Could you check a few things on this model? Use its own coordinates, in mm. Round coordinates to 2 decimals unless told otherwise and drop trailing zeros. Write each loop counter-clockwise with the first axis right and the second up, starting at its lowest first coordinate (ties: lowest second). Pieces come first, ordered by that corner, then holes. Notation, with made-up numbers: (-1, 86) -> (27, 86) arc R11 cw to (27, 93) -> close; hole circle Ø3 at (33.5, -18). An arc over 180 degrees is marked (long way). Answer in a Markdown table with one row per item.
from build123d import *

# Parameters (mm, degrees)
F0_R     = 11
F1_DEPTH = 6.9088
F2_R     = 0.762


with BuildPart() as f1:
    # F0 (on Top) → F1 (new body)
    with BuildSketch(Plane.XY):
        with BuildLine():
            ThreePointArc((-30.12, -12.990381), (-18.81, -8.92943), (-7.5, -12.990381))
            Line((-7.5, -12.990381), (-15, 0))
            Line((-15, 0), (-7.5, 12.990381))
            ThreePointArc((-7.5, 12.990381), (-18.81, 8.92943), (-30.12, 12.990381))
            Line((-30.12, 12.990381), (-22.62, 0))
            Line((-22.62, 0), (-30.12, -12.990381))
        make_face()
        Polygon((22.62, 0), (30.12, -12.990381), (45.12, -12.990381), (52.62, 0), (45.12, 12.990381), (30.12, 12.990381), align=None)
        with Locations((37.62, 0)):
            Circle(F0_R, mode=Mode.SUBTRACT)
        Polygon((-45.12, -12.990381), (-30.12, -12.990381), (-22.62, 0), (-30.12, 12.990381), (-45.12, 12.990381), (-52.62, 0), align=None)
        with Locations((-37.62, 0)):
            Circle(F0_R, mode=Mode.SUBTRACT)
        Polygon((7.5, -12.990381), (15, 0), (7.5, 12.990381), (-7.5, 12.990381), (-15, 0), (-7.5, -12.990381), align=None)
        Circle(F0_R, mode=Mode.SUBTRACT)
        with BuildLine():
            Line((7.5, 12.990381), (15, 0))
            Line((15, 0), (7.5, -12.990381))
            ThreePointArc((7.5, -12.990381), (18.81, -8.92943), (30.12, -12.990381))
            Line((30.12, -12.990381), (22.62, 0))
            Line((22.62, 0), (30.12, 12.990381))
            ThreePointArc((30.12, 12.990381), (18.81, 8.92943), (7.5, 12.990381))
        make_face()
    extrude(amount=F1_DEPTH)

    # F2
    f2_edges = [f1.edges().sort_by_distance(p)[0] for p in [
        (-37.62, 12.990381, 6.9088),
        (-18.81, 8.92943, 6.9088),
        (0, 12.990381, 6.9088),
        (18.81, 8.92943, 6.9088),
        (48.87, 6.495191, 6.9088),
        (48.87, -6.495191, 6.9088),
        (37.62, -12.990381, 6.9088),
        (18.81, -8.92943, 6.9088),
        (0, -12.990381, 6.9088),
        (-37.62, -12.990381, 6.9088),
        (-48.87, 6.495191, 6.9088),
        (-48.87, -6.495191, 6.9088),
        (-18.81, -8.92943, 6.9088),
        (37.62, 12.990381, 6.9088),
        (18.81, -8.92943, 0),
        (0, -12.990381, 0),
        (-18.81, -8.92943, 0),
        (-37.62, -12.990381, 0),
        (-48.87, -6.495191, 0),
        (-48.87, 6.495191, 0),
        (37.62, -12.990381, 0),
        (48.87, -6.495191, 0),
        (52.62, 0, 3.4544),
        (37.62, 12.990381, 0),
        (18.81, 8.92943, 0),
        (0, 12.990381, 0),
        (-18.81, 8.92943, 0),
        (-37.62, 12.990381, 0),
        (48.87, 6.495191, 0),
    ]]
    fillet(f2_edges, radius=F2_R)


solid = f1.part
1) Imagine slicing it at D-D, the plane x = -41.5. Please give me the cut outline in (y, z), plus the area to 3 significant figures.
Findings:
| item | result |
|---|---|
| outline | (-12.99, 0.76) arc R0.76 ccw to (-12.23, 0) -> (-10.29, 0) -> (-10.29, 6.91) -> (-12.23, 6.91) arc R0.76 ccw to (-12.99, 6.15) -> close; (10.29, 0) -> (12.23, 0) arc R0.76 ccw to (12.99, 0.76) -> (12.99, 6.15) arc R0.76 ccw to (12.23, 6.91) -> (10.29, 6.91) -> close |
| area | 36.8 mm^2 |
2) For pin 1 (3 mm diameter, centred on y = 3.5, z = 1.5, fed in from -X); pin 2 (2 mm diameter, centred on x = 8, y = -5, fed in from +Z); pin 3 (2 mm diameter, centred on y = 4, z = 5, fed in from +X), each with a flat end and sliding along its axis, tell me the tip position at first contact or that it passes through.
Findings:
| item | result |
|---|---|
| pin 1 | stops at x = -51.47 |
| pin 2 | passes through |
| pin 3 | stops at x = 50.89 |
3) Please list where these lines run through material, in increasing order: line 1 (Y direction, x = 0, z = 4.25); line 2 (X direction, y = 0.25, z = 1.5); line 3 (X direction, y = 5.75, z = 1.25).
Findings:
| item | result |
|---|---|
| line 1 | y = -12.99 to -11, 11 to 12.99 |
| line 2 | x = -52.48 to -48.62, -26.62 to -11, 11 to 26.62, 48.62 to 52.46 |
| line 3 | x = -49.3 to -47, -28.24 to -9.38, 9.38 to 28.24, 47 to 49.3 |
4) Imagine slicing it at C-C, the plane y = 5.75. Count the separate pieces of the cut face and the enclosed holes in it, plus the area to 3 significant figures.
Findings:
| item | result |
|---|---|
| separate pieces | 4 |
| enclosed holes | 0 |
| area | 292 mm^2 |
5) Thinking about a two-plate mould opening in X: for faces 1 (the face through (47.781, -4.213, 3.406)), 2 (the face through (-46.35, -6.69, 3.41)), 3 (the face through (48.62, -6.49, 0.23)), 4 (the face through (-48.817, 6.586, 3.417)), which applies, +X half, -X half, draft (parallel to the pull), parting line (faces both ways), or undercut?
Findings:
| item | result |
|---|---|
| face 1 | undercut |
| face 2 | undercut |
| face 3 | +X half |
| face 4 | -X half |
6) Imagine slicing it at A-A, the plane x = 37.62. Please give me the cut outline in (y, z), plus the area to 3 significant figures.
Findings:
| item | result |
|---|---|
| outline | (-12.99, 0.76) arc R0.76 ccw to (-12.23, 0) -> (-11, 0) -> (-11, 6.91) -> (-12.23, 6.91) arc R0.76 ccw to (-12.99, 6.15) -> close; (11, 0) -> (12.23, 0) arc R0.76 ccw to (12.99, 0.76) -> (12.99, 6.15) arc R0.76 ccw to (12.23, 6.91) -> (11, 6.91) -> close |
| area | 27.0 mm^2 |
7) Imagine slicing it at B-B, the plane z = 3.75. Please give me the cut outline in (x, y).
Findings:
| item | result |
|---|---|
| outline | (-52.62, 0) -> (-45.12, -12.99) -> (-30.12, -12.99) arc R17.78 cw to (-7.5, -12.99) -> (7.5, -12.99) arc R17.78 cw to (30.12, -12.99) -> (45.12, -12.99) -> (52.4, -0.38) arc R0.76 ccw to (52.4, 0.38) -> (45.12, 12.99) -> (30.12, 12.99) arc R17.78 cw to (7.5, 12.99) -> (-7.5, 12.99) arc R17.78 cw to (-30.12, 12.99) -> (-45.12, 12.99) -> close; hole circle Ø22 at (-37.62, 0); hole circle Ø22 at (0, 0); hole circle Ø22 at (37.62, 0) |
